Geometry check sheet. Reference: the model listing, model coordinates, mm. A direction names the side the tool comes from. Round coordinates to 2 decimals unless told otherwise and drop trailing zeros. Write each loop counter-clockwise with the first axis right and the second up, starting at its lowest first coordinate (ties: lowest second). Pieces come first, ordered by that corner, then holes. Notation, with made-up numbers: M 17,-26.5 L 35,-26.5 A20 cw 35,-20.5 Z; hole C 74,54 d5. An arc over 180 degrees is marked long. One line per item, written item: value. Start each with the question number.
1. Section check C-C (x = 139). Record the boundary of the cut face in (y, z).
2. Release check for a two-part mould opening along Y. For faces 3 (the flat face through (-1, 0, -3)), 4 (the flat face through (-1, -38, 203.2)), 5 (the flat face through (-152.4, -38, 12)) record: pulls with the +Y half, pulls with the -Y half, needs draft (parallel to the pull), parting line crosses it, or undercut.
3. Scan lines: probe 1 along X at (y, z) = (-46, -159.5); probe 2 along X at (y, z) = (-4, 78); probe 3 along Z at (x, y) = (-114.5, -20.5). Record each from-to range of solid material in increasing order. Write a range as [from, to].
4. Section check B-B (z = 102). Record the boundary of the cut face in (x, y).
5. Section check A-A (y = -45.5). Record the boundary of the cut face in (x, z).
6. Depth check by flat-ended pin: P1, Ø0.8, axis at x = -154, y = -10, coming from the +Z side; P2, Ø4, axis at x = 156, y = -37.5, coming from the +Z side; P3, Ø12, axis at y = -41.5, z = 34.5, coming from the -X side. Enter the tip coordinate at first touch or a pass-through.
7. Access from +Z, -Z, +X, -X, +Y, -Y to the whole of each face (thin tool, end or side, straight path). Record for faces 1 (the flat face through (-1, -76.2, -3)), 2 (the flat face through (152.4, -38, 36)).
from build123d import *

# Parameters (mm, degrees)
F0_W     = 304.8
F0_H     = 406.4
F1_DEPTH = 76.2
F2_SIZE  = 50.8
F3_W     = 25.4
F3_H     = 101.6
F4_DEPTH = 2.54
F5_W     = 76.2
F5_H     = 127
F6_DEPTH = 5.08


with BuildPart() as f1:
    # F0 (on Front) → F1 (new body)
    with BuildSketch(Plane.XZ):
        Rectangle(F0_W, F0_H)
    extrude(amount=F1_DEPTH)

    # F2
    f2_edges = [f1.edges().sort_by_distance(p)[0] for p in [
        (-152.4, -38.1, 203.2),
        (152.4, -38.1, 203.2),
    ]]
    chamfer(f2_edges, length=F2_SIZE)

    # F3 (on face) → F4 (join)
    with BuildSketch(Plane(origin=(-152.4, 0, 0), x_dir=(0, -1, 0), z_dir=(-1, 0, 0))):
        with Locations((12.7, -152.4)):
            Rectangle(F3_W, F3_H)
        with Locations((63.5, -152.4)):
            Rectangle(F3_W, F3_H)
    extrude(amount=F4_DEPTH)

    # F5 (on face) → F6 (join)
    with BuildSketch(Plane.YZ.offset(152.4)):
        with Locations((-38.1, -139.7)):
            Rectangle(F5_W, F5_H)
    extrude(amount=F6_DEPTH)


solid = f1.part
Result sheet:
1. outline: M -76.2,-203.2 L 0,-203.2 L 0,165.8 L -76.2,165.8 Z
2. face 3: pulls with the +Y half
2. face 4: needs draft
2. face 5: undercut
3. probe 1: x = [-152.4, 157.48]
3. probe 2: x = [-152.4, 152.4]
3. probe 3: z = [-203.2, 190.3]
4. outline: M -152.4,-76.2 L 152.4,-76.2 L 152.4,0 L -152.4,0 Z
5. outline: M -152.4,-203.2 L 157.48,-203.2 L 157.48,-76.2 L 152.4,-76.2 L 152.4,152.4 L 101.6,203.2 L -101.6,203.2 L -152.4,152.4 Z
6. P1: stops at z = -101.6
6. P2: stops at z = -76.2
6. P3: stops at x = -152.4
7. face 1: +Z, -Z, +X, -X, -Y
7. face 2: +Z, +X, +Y, -Y
